CAD build for the part. Positions are in the model's coordinates, mm. A direction names the side the tool comes from. Give positions to 0.01 mm unless a question says otherwise; leave off trailing zeros. Write each loop counter-clockwise with the first axis right and the second up, starting at its lowest first coordinate (ties: lowest second). Pieces come first, ordered by that corner, then holes. Notation, with made-up numbers: (-6.5, -34) - (5.5, -34) arc R22 cw to (5.5, -9) - close; hole circle Ø7 at (54, -17). An arc over 180 degrees is marked (long way). Write item = value, one per line. Start each with the question number.
```python
from build123d import *

# Parameters (mm, degrees)
F0_R     = 7.5
F1_DEPTH = 2
F3_DEPTH = 2
F5_DEPTH = 3


with BuildPart() as f1:
    # F0 (on Top) → F1 (new body)
    with BuildSketch(Plane.XY):
        Circle(F0_R)
    extrude(amount=F1_DEPTH)

    # F2 (on face) → F3 (join)
    with BuildSketch(Plane.XY.offset(2)):
        with BuildLine():
            Line((0, -1.738777), (0, 5.421451))
            ThreePointArc((0, 5.421451), (-1.329954, 4.285908), (-0.416891, 2.794415))
            Line((-0.416891, 2.794415), (-0.416891, 1.635802))
            Line((-0.416891, 1.635802), (-1.318156, 1.635802))
            Line((-1.318156, 1.635802), (-2.654623, 2.80521))
            Line((-2.654623, 2.80521), (-3.214125, 5.707625))
            Line((-3.214125, 5.707625), (-4.179397, 5.521548))
            Line((-4.179397, 5.521548), (-3.524426, 2.123883))
            Line((-3.524426, 2.123883), (-1.78592, 0.80051))
            Line((-1.78592, 0.80051), (-1.012103, -1.049922))
            Line((-1.012103, -1.049922), (-2.086625, -3.242302))
            Line((-2.086625, -3.242302), (-3.084522, -6.387633))
            Line((-3.084522, -6.387633), (-1.932593, -6.753098))
            Line((-1.932593, -6.753098), (-0.980974, -3.669764))
            Line((-0.980974, -3.669764), (0, -1.738777))
        make_face()
        with BuildLine():
            ThreePointArc((0.416891, 2.794415), (1.329954, 4.285908), (0, 5.421451))
            Line((0, 5.421451), (0, -1.738777))
            Line((0, -1.738777), (0.980974, -3.669764))
            Line((0.980974, -3.669764), (1.932593, -6.753098))
            Line((1.932593, -6.753098), (3.084522, -6.387633))
            Line((3.084522, -6.387633), (2.086625, -3.242302))
            Line((2.086625, -3.242302), (1.012103, -1.049922))
            Line((1.012103, -1.049922), (1.78592, 0.80051))
            Line((1.78592, 0.80051), (3.524426, 2.123883))
            Line((3.524426, 2.123883), (4.179397, 5.521548))
            Line((4.179397, 5.521548), (3.214125, 5.707625))
            Line((3.214125, 5.707625), (2.654623, 2.80521))
            Line((2.654623, 2.80521), (1.318156, 1.635802))
            Line((1.318156, 1.635802), (0.416891, 1.635802))
            Line((0.416891, 1.635802), (0.416891, 2.794415))
        make_face()
    extrude(amount=F3_DEPTH)

    # F4 (on face) → F5 (join)
    with BuildSketch(Plane.XY.offset(2)):
        Polygon((-2.225088, 5.01617), (-5.260212, 4.431086), (-5.012016, 3.632387), (-2.067746, 4.199957), align=None)
        Polygon((-0.703037, -5.554148), (-3.730533, -4.513447), (-3.987216, -5.282778), (-0.980974, -6.34256), align=None)
        Polygon((5.012016, 3.632387), (5.260212, 4.431086), (2.225088, 5.01617), (2.067746, 4.199957), align=None)
        Polygon((3.987216, -5.282778), (3.730533, -4.513447), (0.703037, -5.554148), (0.980974, -6.34256), align=None)
    extrude(amount=F5_DEPTH)


solid = f1.part
```
1. Cut at B-B (z = 0.45). Give the cut face in (x, y).
2. Tool access for faces 5 (the flat face through (-4, 4, 5)), 6 (the flat face through (1.557, -2.161, 2.986)), 7 (the flat face through (-3.13, 5.28, 2.99)), 8 (the flat face through (2.775, 3.432, 2.986)), 9 (the flat face through (-1.404, -0.112, 2.986)): list every direction of +Z, -Z, +X, -X, +Y, -Y with a clear straight run to the whole face (end or side of a thin tool).
3. Cut at C-C (x = -6). Give the cut face in (y, z).
4. Mould opens along X. For faces 1 (the cylindrical face through (-7.493, 0.33, 0.986)), 2 (the flat face through (3.6, 5.2, 4)), 3 (the flat face through (-1.977, 2.212, 2.986)), 4 (the flat face through (-2.517, -6.568, 2.986)) say: +X half, -X half, draft (parallel to the pull), parting line (faces both ways), or undercut.
5. Wall check: line 1 along Z through (x, y) = (-5, 5); line 2 along X through (y, z) = (-0.25, 1.5); line 3 along Z through (x, y) = (2.25, -6.25). Give the ranges that are in metal, low to high.
6. Cut at A-A (y = 0). Give the cut face in (x, z).
7. Pin check, flat tips, straight feed: pin 1 Ø1.5 at (x, y) = (6, 0.5) entering from +Z; pin 2 Ø2.5 at (x, y) = (0.5, 0) entering from +Z; pin 3 Ø0.5 at (x, z) = (-1, 2.5) entering from +Y. Stop position of each tip, or through.
Output:
q1.outline = circle Ø15 at (0, 0)
q2.face_5 = +Z, +X, -X, +Y, -Y
q2.face_6 = +Z, +X
q2.face_7 = +Z, +Y
q2.face_8 = +Z
q2.face_9 = +Z, -X
q3.outline = (-4.5, 0) - (4.5, 0) - (4.5, 2) - (-4.5, 2) - close
q4.face_1 = parting line
q4.face_2 = draft
q4.face_3 = undercut
q4.face_4 = -X half
q5.line_1 = 0 to 2
q5.line_2 = -7.5 to 7.5
q5.line_3 = 0 to 4
q6.outline = (-7.5, 0) - (7.5, 0) - (7.5, 2) - (1.45, 2) - (1.45, 4) - (-1.45, 4) - (-1.45, 2) - (-7.5, 2) - close
q7.pin_1 = 2
q7.pin_2 = 4
q7.pin_3 = 5.19
